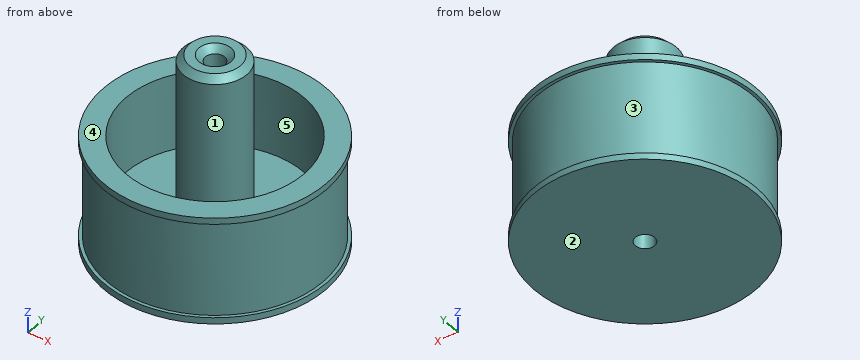
```python
from build123d import *

# Parameters (mm, degrees)
F0_R      = 17.5
F1_DEPTH  = 1
F2_R      = 17
F3_DEPTH  = 15
F4_R      = 17.5
F5_DEPTH  = 1
F6_R      = 14
F7_DEPTH  = 12
F8_R      = 5
F9_DEPTH  = 25
F10_R     = 1.525
F11_DEPTH = 30
F12_SIZE  = 1


with BuildPart() as f1:
    # F0 (on Top) → F1 (new body)
    with BuildSketch(Plane.XY):
        Circle(F0_R)
    extrude(amount=F1_DEPTH)

    # F2 (on face) → F3 (join)
    with BuildSketch(Plane.XY.offset(1)):
        Circle(F2_R)
    extrude(amount=F3_DEPTH)

    # F4 (on face) → F5 (join)
    with BuildSketch(Plane.XY.offset(16)):
        Circle(F4_R)
    extrude(amount=F5_DEPTH)

    # F6 (on face) → F7 (cut)
    with BuildSketch(Plane.XY.offset(17)):
        Circle(F6_R)
    extrude(amount=-F7_DEPTH, mode=Mode.SUBTRACT)

    # F8 (on face) → F9 (join)
    with BuildSketch(Plane.XY.offset(5)):
        Circle(F8_R)
    extrude(amount=F9_DEPTH)

    # F10 (on face) → F11 (cut, through all)
    with BuildSketch(Plane.XY.offset(30)):
        Circle(F10_R)
    extrude(amount=-F11_DEPTH, mode=Mode.SUBTRACT)

    # F12
    f12_edges = [f1.edges().sort_by_distance(p)[0] for p in [
        (-1.525, 0, 30),
        (-5, 0, 30),
    ]]
    chamfer(f12_edges, length=F12_SIZE)


solid = f1.part
```
Check sheet for the modelled part. Datum: model origin and axes. Units: mm. Face numbers are marked on the shaded views. A direction names the side the tool comes from. Give positions to 0.01 mm unless a question says otherwise; leave off trailing zeros. Write each loop counter-clockwise with the first axis right and the second up, starting at its lowest first coordinate (ties: lowest second). Pieces come first, ordered by that corner, then holes. Notation, with made-up numbers: (22.25, 14) - (71.25, 14) arc R21 ccw to (71.25, 24) - close; hole circle Ø4 at (-12.75, 12). An arc over 180 degrees is marked (long way). Answer as a JSON object with one key per item and string values. Group by question number.
1) Access from +Z, -Z, +X, -X, +Y, -Y to the whole of each face (thin tool, end or side, straight path). Record for the marked faces 1 and 2.
2) Sectioned sample at C-C (z = 4). Record the cut outline in (x, y) (3 decimals), then the cut area to 3 significant figures.
3) Thickness scan on probe 1 along Y at (x, z) = (0, 14.25) (3 decimals); probe 2 along X at (y, z) = (-3.5, 10); probe 3 along Y at (x, z) = (-1, 12). Record the ranges inside material, lowest first. Write a range as from..to.
4) Depth check by flat-ended pin: P1, Ø1, axis at x = -13, y = -10, coming from the -Z side; P2, Ø3, axis at y = 6.5, z = 10.5, coming from the -X side; P3, Ø6, axis at x = 9.5, z = 10.5, coming from the +Y side; P4, Ø1, axis at y = 4, z = 15, coming from the -X side. Enter the tip coordinate at first touch or a pass-through.
5) Sectioned sample at B-B (z = 12). Record the cut outline in (x, y) (3 decimals).
6) Release check for a two-part mould opening along Y. For the marked faces 3, 4 and 5 record: pulls with the +Y half, pulls with the -Y half, needs draft (parallel to the pull), parting line crosses it, or undercut.
7) Sectioned sample at A-A (x = 0). Record the cut outline in (y, z) (3 decimals).
8) Sectioned sample at D-D (y = 6). Record the cut outline in (x, z), then the cut area to 3 significant figures.
Geometry results:
{
 "1": {"face 1": "+Z", "face 2": "-Z, +X, -X, +Y, -Y"},
 "2": {"outline": "circle Ø34 at (0, 0); hole circle Ø3.05 at (0, 0)", "area": "901 mm^2"},
 "3": {"probe 1": "y = -17..-14, -5..-1.525, 1.525..5, 14..17", "probe 2": "x = -16.64..-13.56, -3.57..3.57, 13.56..16.64", "probe 3": "y = -16.97..-13.96, -4.9..-1.15, 1.15..4.9, 13.96..16.97"},
 "4": {"P1": "stops at z = 0", "P2": "stops at x = -16.25", "P3": "stops at y = 15.71", "P4": "stops at x = -16.64"},
 "5": {"outline": "circle Ø34 at (0, 0); circle Ø10 at (0, 0); hole circle Ø28 at (0, 0); hole circle Ø3.05 at (0, 0)"},
 "6": {"face 3": "parting line crosses it", "face 4": "needs draft", "face 5": "undercut"},
 "7": {"outline": "(-17.5, 0) - (-1.525, 0) - (-1.525, 29) - (-2.525, 30) - (-4, 30) - (-5, 29) - (-5, 5) - (-14, 5) - (-14, 17) - (-17.5, 17) - (-17.5, 16) - (-17, 16) - (-17, 1) - (-17.5, 1) - close; (1.525, 0) - (17.5, 0) - (17.5, 1) - (17, 1) - (17, 16) - (17.5, 16) - (17.5, 17) - (14, 17) - (14, 5) - (5, 5) - (5, 29) - (4, 30) - (2.525, 30) - (1.525, 29) - close"},
 "8": {"outline": "(-16.44, 0) - (16.44, 0) - (16.44, 1) - (15.91, 1) - (15.91, 16) - (16.44, 16) - (16.44, 17) - (12.65, 17) - (12.65, 5) - (-12.65, 5) - (-12.65, 17) - (-16.44, 17) - (-16.44, 16) - (-15.91, 16) - (-15.91, 1) - (-16.44, 1) - close", "area": "239 mm^2"}
}
